from build123d import *

# Parameters (mm, degrees)
SKETCH2_R            = 5.5
BOSS_EXTRUDE1_DEPTH  = 19.05
M3_CLEARANCE_HOLE1_D = 3.4
CIRPATTERN1_COUNT    = 4
FILLET1_R            = 10
M3_CLEARANCE_HOLE2_D = 3.4
CIRPATTERN2_COUNT    = 4
M3_CLEARANCE_HOLE3_D = 3.4
CIRPATTERN3_COUNT    = 4


with BuildPart() as part:
    # Sketch2 → Boss-Extrude1 (new body)
    with BuildSketch(Plane(origin=(0, 0, 0), x_dir=(1, 0, 0), z_dir=(0, 1, 0))):
        Polygon((0, 0), (467.5, 0), (467.5, 510), (317.652811453, 510), (317.652811453, 535), (149.847188547, 535), (149.847188547, 510), (0, 510), align=None)
        with Locations(Location((233.75, 500, 0), (0, 0, 90))):
            Circle(SKETCH2_R, mode=Mode.SUBTRACT)
        with Locations(Location((20, 40, 0), (0, 0, 90))):
            Circle(SKETCH2_R, mode=Mode.SUBTRACT)
        with Locations(Location((447.5, 40, 0), (0, 0, 90))):
            Circle(SKETCH2_R, mode=Mode.SUBTRACT)
    extrude(amount=BOSS_EXTRUDE1_DEPTH)

    # M3 Clearance Hole1 (through all)
    with Locations(Plane(origin=(225.75, 19.05, -500), x_dir=(0, 0, 1), z_dir=(0, 1, 0))):
        with Locations((0, 0)):
            m3_clearance_hole1 = Hole(M3_CLEARANCE_HOLE1_D / 2)

    # CirPattern1: M3 Clearance Hole1 ×4 about axis
    cirpattern1_axis = Axis((233.75, 0, -500), (0, 1, 0))
    for i in range(1, CIRPATTERN1_COUNT):
        add(m3_clearance_hole1.rotate(cirpattern1_axis, i * 360 / CIRPATTERN1_COUNT), mode=Mode.SUBTRACT)

    # Fillet1
    fillet1_edges = [part.edges().sort_by_distance(p)[0] for p in [
        (149.847188547, 9.525, -510),
        (149.847188547, 9.525, -535),
        (317.652811453, 9.525, -535),
        (317.652811453, 9.525, -510),
    ]]
    fillet(fillet1_edges, radius=FILLET1_R)

    # M3 Clearance Hole2 (through all)
    with Locations(Plane(origin=(20, 19.05, -48), x_dir=(0, 0, 1), z_dir=(0, 1, 0))):
        with Locations((0, 0)):
            m3_clearance_hole2 = Hole(M3_CLEARANCE_HOLE2_D / 2)

    # CirPattern2: M3 Clearance Hole2 ×4 about axis
    cirpattern2_axis = Axis((20, 0, -40), (0, 1, 0))
    for i in range(1, CIRPATTERN2_COUNT):
        add(m3_clearance_hole2.rotate(cirpattern2_axis, i * 360 / CIRPATTERN2_COUNT), mode=Mode.SUBTRACT)

    # M3 Clearance Hole3 (through all)
    with Locations(Plane(origin=(447.5, 19.05, -48), x_dir=(0, 0, 1), z_dir=(0, 1, 0))):
        with Locations((0, 0)):
            m3_clearance_hole3 = Hole(M3_CLEARANCE_HOLE3_D / 2)

    # CirPattern3: M3 Clearance Hole3 ×4 about axis
    cirpattern3_axis = Axis((447.5, 0, -40), (0, 1, 0))
    for i in range(1, CIRPATTERN3_COUNT):
        add(m3_clearance_hole3.rotate(cirpattern3_axis, i * 360 / CIRPATTERN3_COUNT), mode=Mode.SUBTRACT)


solid = part.part
The listing builds one solid part. Answer for the finished solid, in the listing's coordinates (mm). A direction names the side the tool comes from. Give positions to 0.01 mm unless a question says otherwise; leave off trailing zeros. Write each loop counter-clockwise with the first axis right and the second up, starting at its lowest first coordinate (ties: lowest second). Pieces come first, ordered by that corner, then holes. Notation, with made-up numbers: (-17, 9.25) - (27, 9.25) arc R37 cw to (27, 46.25) - close; hole circle Ø9 at (22, -20.75). An arc over 180 degrees is marked (long way). Use a Markdown table: item, result.
1. Section B-B on x = 126.5 is taken. Write down the section's boundary in (y, z), plus the area to 3 significant figures.
Values follow:
| item | result |
|---|---|
| outline | (0, -510) - (19.05, -510) - (19.05, 0) - (0, 0) - close |
| area | 9,720 mm² |
2. A tool of negligible diameter and unlimited length cuts with its end or side. For faces 5 (the flat face through (71, 9, -510)), 6 (the flat face through (467.5, 9, -251)), 7 (the flat face through (399, 9, -510)), from which of +Z, -Z, +X, -X, +Y, -Y can it reach the whole face along a straight path? Write none if from no direction.
Values follow:
| item | result |
|---|---|
| face 5 | -Z, -X, +Y, -Y |
| face 6 | +Z, -Z, +X, +Y, -Y |
| face 7 | -Z, +X, +Y, -Y |
3. Each of these flat-tipped pins is pushed along its axis until it touches: P1, Ø2.5, axis at y = 8, z = -523, coming from the -X side; P2, Ø5.5, axis at x = 416.5, y = 10.5, coming from the -Z side. Where does it stop, or does it pass through?
Values follow:
| item | result |
|---|---|
| P1 | stops at x = 149.85 |
| P2 | stops at z = -510 |
4. For a pull along Z with two mould halves and no side action, classify faces 1 (the cylindrical face through (452.87, 9.39, -38.81)), 2 (the flat face through (235, 9, -535)), 3 (the flat face through (230, 0, -271)), 4 (the flat face through (230, 9, 0)) as released by +Z, released by -Z, zero draft, split by the parting line, or undercut.
Values follow:
| item | result |
|---|---|
| face 1 | undercut |
| face 2 | released by -Z |
| face 3 | zero draft |
| face 4 | released by +Z |
5. Section A-A on y = 6.25 is taken. Count the separate pieces of the cut face and the enclosed holes in it, plus the area to 3 significant figures.
Values follow:
| item | result |
|---|---|
| separate pieces | 1 |
| enclosed holes | 15 |
| area | 242,000 mm² |
6. Find the intervals of material crossed by probe 1 along X at (y, z) = (5, -500); probe 2 along Z at (x, y) = (447.5, 15.25); probe 3 along X at (y, z) = (10.75, -32), in increasing order. Write a range as from..to.
Values follow:
| item | result |
|---|---|
| probe 1 | x = 0..224.05, 227.45..228.25, 239.25..240.05, 243.45..467.5 |
| probe 2 | z = -510..-49.7, -46.3..-45.5, -34.5..-33.7, -30.3..0 |
| probe 3 | x = 0..18.3, 21.7..445.8, 449.2..467.5 |
